```python
from build123d import *

# Parameters (mm, degrees)
F1_DEPTH = 0.79375


# Not quite as in the source:
# - a length typed as a fraction of an inch, garbled in the dataset ("3 / 203.2 mm" for 3/8 in), is restored


with BuildPart() as f1:
    # F0 (on Top) → F1 (new body)
    with BuildSketch(Plane.XY):
        with BuildLine():
            ThreePointArc((0, 3.5875), (-0.4649679849, 2.4649679849), (-1.5875, 2))
            Line((-1.5875, 2), (-48.4125, 2))
            ThreePointArc((-48.4125, 2), (-49.5350320151, 2.4649679849), (-50, 3.5875))
            Line((-50, 3.5875), (-50, 5))
            Line((-50, 5), (-52, 5))
            Line((-52, 5), (-52, 3.5875))
            ThreePointArc((-52, 3.5875), (-52.4649679849, 2.4649679849), (-53.5875, 2))
            Line((-53.5875, 2), (-54, 2))
            Line((-54, 2), (-54, -2))
            Line((-54, -2), (-53.5875, -2))
            ThreePointArc((-53.5875, -2), (-52.4649679849, -2.4649679849), (-52, -3.5875))
            Line((-52, -3.5875), (-52, -5))
            Line((-52, -5), (-50, -5))
            Line((-50, -5), (-50, -3.5875))
            ThreePointArc((-50, -3.5875), (-49.5350320151, -2.4649679849), (-48.4125, -2))
            Line((-48.4125, -2), (-1.5875, -2))
            ThreePointArc((-1.5875, -2), (-0.4649679849, -2.4649679849), (0, -3.5875))
            Line((0, -3.5875), (0, -5))
            Line((0, -5), (2, -5))
            Line((2, -5), (2, 5))
            Line((2, 5), (0, 5))
            Line((0, 5), (0, 3.5875))
        make_face()
    extrude(amount=F1_DEPTH)


solid = f1.part
```
Part model, mm, in its own coordinate system. A direction names the side the tool comes from. Coordinates: 2 decimals unless noted, no trailing zeros. Loops run counter-clockwise (first coordinate to the right, second up) from the corner with the lowest first, then second, coordinate; pieces in that order, holes last. Notation, with made-up numbers: (21, 23) - (43, 23) arc R38 ccw to (43, 62) - close; hole circle Ø8 at (75.25, 10). An arc over 180 degrees is marked (long way). Write item = value, one per line. Start each with the question number.
Item 1: Cut at B-B, the plane y = 2.5. Give the cut face in (x, z), and give its area (3 significant figures).
Item 2: Cut at D-D, the plane x = -49.5. Give the cut face in (y, z).
Item 3: Wall check: L1, parallel to X at y = -4, z = 0.2; L2, parallel to Y at x = -12.5, z = 0.5; L3, parallel to X at y = -2.25, z = 0.4. Give the ranges that are in metal, low to high. Write a range as from..to.
Item 4: Cut at A-A, the plane z = 0.25. Give the cut face in (x, y) (1 decimal), and give its area (3 significant figures).
Item 5: 3-axis set-ups, long thin cutter, end or side, ignore diameter. For faces 1 (the cylindrical face through (-49.52, 2.45, 0.39)), 2 (the cylindrical face through (-52.48, -2.45, 0.39)): which of +Z, -Z, +X, -X, +Y, -Y reach the whole face in a straight line?
Item 6: Cut at C-C, the plane x = -28.5. Give the cut face in (y, z), and give its area (4 significant figures).
Item 7: Mould opens along X. For faces 3 (the flat face through (-33, 0, 0.794)), 4 (the cylindrical face through (-49.55, -2.48, 0.39)), 5 (the cylindrical face through (-52.45, 2.48, 0.39)), 6 (the cylindrical face through (-0.48, -2.45, 0.39)) say: released by +X, released by -X, zero draft, split by the parting line, or undercut.
The answers:
q1.outline = (-52.43, 0) - (-49.57, 0) - (-49.57, 0.79) - (-52.43, 0.79) - close; (-0.43, 0) - (2, 0) - (2, 0.79) - (-0.43, 0.79) - close
q1.area = 4.20 mm2
q2.outline = (-2.43, 0) - (2.43, 0) - (2.43, 0.79) - (-2.43, 0.79) - close
q3.L1 = -52..-50, 0..2
q3.L2 = -2..2
q3.L3 = -52.73..-49.27, -0.73..2
q4.outline = (-54, -2) - (-53.6, -2) arc R1.6 cw to (-52, -3.6) - (-52, -5) - (-50, -5) - (-50, -3.6) arc R1.6 cw to (-48.4, -2) - (-1.6, -2) arc R1.6 cw to (0, -3.6) - (0, -5) - (2, -5) - (2, 5) - (0, 5) - (0, 3.6) arc R1.6 cw to (-1.6, 2) - (-48.4, 2) arc R1.6 cw to (-50, 3.6) - (-50, 5) - (-52, 5) - (-52, 3.6) arc R1.6 cw to (-53.6, 2) - (-54, 2) - close
q4.area = 251 mm2
q5.face_1 = +Z, -Z, +Y
q5.face_2 = +Z, -Z, -X, -Y
q6.outline = (-2, 0) - (2, 0) - (2, 0.79) - (-2, 0.79) - close
q6.area = 3.175 mm2
q7.face_3 = zero draft
q7.face_4 = undercut
q7.face_5 = released by -X
q7.face_6 = undercut
